Verification items for the finished model (mm, model axes). A direction names the side the tool comes from. Give positions to 0.01 mm unless a question says otherwise; leave off trailing zeros. Order: outer loops, then holes, each group sorted by start corner. A loop starts at its lowest first (then second) coordinate and runs counter-clockwise, first axis right, second up.
Autodesk Inventor part; units mm, degrees
ref_plane "YZ Plane" through (0, 0, 0) normal (1, 0, 0) x (0, 1, 0)
ref_plane "XZ Plane" through (0, 0, 0) normal (0, 1, 0) x (-1, 0, 0)
ref_plane "XY Plane" through (0, 0, 0) normal (0, 0, 1) x (1, 0, 0)
sketch "スケッチ1" plane through (0, 0, 0) normal (0, 0, 1) x (1, 0, 0)
  circle A0 centre (20, -42) radius 1
  circle A1 centre (4, -42) radius 1
  circle A2 centre (20, -6) radius 1
  circle A3 centre (20, -42) radius 1.1
  line L0 (22.5, -78.2) -> (22.5, -32.2)
  circle A4 centre (20, -42) radius 2.5
  circle A5 centre (20, -6) radius 2.5
  circle A6 centre (20, -6) radius 1.1
  circle A7 centre (4, -42) radius 1.1
  circle A8 centre (4, -42) radius 2.5
  line L1 (-8, -45.7) -> (-8, -64.7)
  line L2 (-8, -44.5) -> (-8, -39.5)
  line L3 (17.5, -42) -> (17.5, -6)
  line L4 (20, -39.5) -> (-8, -39.5)
  line L5 (20, -44.5) -> (4, -44.5)
  line L6 (4, -44.5) -> (-8, -44.5)
  line L7 (24, -24.4) -> (24, -30)
  line L8 (24, -32.2) -> (22.5, -32.2)
  line L9 (24, -22.2) -> (22.5, -22.2)
  line L10 (24, -32.2) -> (22.5, -32.2)
  line L11 (22.5, -32.2) -> (22.5, -22.2)
  line L12 (22.5, -22.2) -> (24, -22.2)
  line L13 (24, -22.2) -> (24, -32.2)
  line L14 (22.5, -22.2) -> (22.5, -6)
  line L15 (2, -43.5) -> (2, -4.5)
  arc A9 (2, -43.5) -> (2.5, -44) centre (2.5, -43.5) ccw
  line L16 (21.5, -44) -> (2.5, -44)
  arc A10 (21.5, -44) -> (22, -43.5) centre (21.5, -43.5) ccw
  line L17 (22, -4.5) -> (22, -43.5)
  arc A11 (22, -4.5) -> (21.5, -4) centre (21.5, -4.5) ccw
  line L18 (2.5, -4) -> (21.5, -4)
  arc A12 (2.5, -4) -> (2, -4.5) centre (2.5, -4.5) ccw
  line L19 (18.4286, -23.8214) -> (18.4286, -30.1786)
  line L20 (18.4286, -30.1786) -> (14.5714, -30.1786)
  line L21 (14.5714, -30.1786) -> (14.5714, -23.8214)
  line L22 (14.5714, -23.8214) -> (18.4286, -23.8214)
  circle A13 centre (12, -31.4) radius 1.1519
  line L23 (5.5714, -23.8214) -> (9.4286, -23.8214)
  line L24 (9.4286, -23.8214) -> (9.4286, -30.1786)
  line L25 (9.4286, -30.1786) -> (5.5714, -30.1786)
  line L26 (5.5714, -30.1786) -> (5.5714, -23.8214)
  circle A14 centre (20, -6) radius 1.8131
  circle A15 centre (4, -6) radius 1.8131
  circle A16 centre (20, -42) radius 1.8131
  circle A17 centre (4, -42) radius 1.8131
  arc A18 (18.25, -12.4893) -> (5.75, -12.5) centre (12, -12.5) ccw
  arc A19 (18.5, -12.25) -> (18.2502, -12.4893) centre (18.5, -12.5) ccw
  line L27 (18.5, -12.25) -> (20.25, -12.25)
  arc A20 (20.25, -12.75) -> (20.25, -12.25) centre (20.25, -12.5) ccw
  line L28 (20.25, -12.75) -> (18.5, -12.75)
  arc A21 (18.25, -12.5) -> (18.5, -12.75) centre (18.5, -12.5) ccw
  arc A22 (17.7742, -14.8918) -> (18.25, -12.5) centre (12, -12.5) ccw
  arc A23 (18.1009, -14.7565) -> (17.7742, -14.8918) centre (18.0052, -14.9874) ccw
  line L29 (18.1009, -14.7565) -> (19.7177, -15.4262)
  arc A24 (19.5263, -15.8881) -> (19.7177, -15.4262) centre (19.622, -15.6571) ccw
  line L30 (19.5263, -15.8881) -> (17.9095, -15.2184)
  arc A25 (17.7742, -14.8918) -> (17.9095, -15.2184) centre (18.0052, -14.9874) ccw
  arc A26 (16.4194, -16.9194) -> (17.7742, -14.8918) centre (12, -12.5) ccw
  arc A27 (16.773, -16.9194) -> (16.4194, -16.9194) centre (16.5962, -17.0962) ccw
  line L31 (16.773, -16.9194) -> (18.0104, -18.1569)
  arc A28 (17.6569, -18.5104) -> (18.0104, -18.1569) centre (17.8336, -18.3336) ccw
  line L32 (17.6569, -18.5104) -> (16.4194, -17.273)
  arc A29 (16.4194, -16.9194) -> (16.4194, -17.273) centre (16.5962, -17.0962) ccw
  arc A30 (14.3918, -18.2742) -> (16.4194, -16.9194) centre (12, -12.5) ccw
  arc A31 (14.7184, -18.4095) -> (14.3918, -18.2742) centre (14.4874, -18.5052) ccw
  line L33 (14.7184, -18.4095) -> (15.3881, -20.0263)
  arc A32 (14.9262, -20.2177) -> (15.3881, -20.0263) centre (15.1571, -20.122) ccw
  line L34 (14.9262, -20.2177) -> (14.2565, -18.6009)
  arc A33 (14.3918, -18.2742) -> (14.2565, -18.6009) centre (14.4874, -18.5052) ccw
  arc A34 (12, -18.75) -> (14.3918, -18.2742) centre (12, -12.5) ccw
  arc A35 (12.25, -19) -> (12, -18.75) centre (12, -19) ccw
  line L35 (12.25, -19) -> (12.25, -20.75)
  arc A36 (11.75, -20.75) -> (12.25, -20.75) centre (12, -20.75) ccw
  line L36 (11.75, -20.75) -> (11.75, -19)
  arc A37 (12, -18.75) -> (11.75, -19) centre (12, -19) ccw
  arc A38 (9.6082, -18.2742) -> (12, -18.75) centre (12, -12.5) ccw
  arc A39 (9.7435, -18.6009) -> (9.6082, -18.2742) centre (9.5126, -18.5052) ccw
  line L37 (9.7435, -18.6009) -> (9.0738, -20.2177)
  arc A40 (8.6119, -20.0263) -> (9.0738, -20.2177) centre (8.8429, -20.122) ccw
  line L38 (8.6119, -20.0263) -> (9.2816, -18.4095)
  arc A41 (9.6082, -18.2742) -> (9.2816, -18.4095) centre (9.5126, -18.5052) ccw
  arc A42 (7.5806, -16.9194) -> (9.6082, -18.2742) centre (12, -12.5) ccw
  arc A43 (7.5806, -17.273) -> (7.5806, -16.9194) centre (7.4038, -17.0962) ccw
  line L39 (7.5806, -17.273) -> (6.3431, -18.5104)
  arc A44 (5.9896, -18.1569) -> (6.3431, -18.5104) centre (6.1664, -18.3336) ccw
  line L40 (5.9896, -18.1569) -> (7.227, -16.9194)
  arc A45 (7.5806, -16.9194) -> (7.227, -16.9194) centre (7.4038, -17.0962) ccw
  arc A46 (6.2258, -14.8918) -> (7.5806, -16.9194) centre (12, -12.5) ccw
  arc A47 (6.0905, -15.2184) -> (6.2258, -14.8918) centre (5.9948, -14.9874) ccw
  line L41 (6.0905, -15.2184) -> (4.4737, -15.8881)
  arc A48 (4.2823, -15.4262) -> (4.4737, -15.8881) centre (4.378, -15.6571) ccw
  line L42 (4.2823, -15.4262) -> (5.8991, -14.7565)
  arc A49 (6.2258, -14.8918) -> (5.8991, -14.7565) centre (5.9948, -14.9874) ccw
  arc A50 (5.75, -12.5) -> (6.2258, -14.8918) centre (12, -12.5) ccw
  arc A51 (5.5, -12.75) -> (5.75, -12.5) centre (5.5, -12.5) ccw
  line L43 (5.5, -12.75) -> (3.75, -12.75)
  arc A52 (3.75, -12.25) -> (3.75, -12.75) centre (3.75, -12.5) ccw
  line L44 (3.75, -12.25) -> (5.5, -12.25)
  arc A53 (5.75, -12.5) -> (5.5, -12.25) centre (5.5, -12.5) ccw
  line L45 (18.9286, -30.6786) -> (18.9286, -23.3214)
  line L46 (18.9286, -23.3214) -> (14.0714, -23.3214)
  line L47 (14.0714, -23.3214) -> (14.0714, -30.6786)
  line L48 (14.0714, -30.6786) -> (18.9286, -30.6786)
  circle A54 centre (22.5, -21.1) radius 1.1
  circle A55 centre (22.5, -33.3) radius 1.1
  circle A56 centre (-9, -42) radius 1.1
  circle A57 centre (12, -12.5) radius 6.25
  circle A58 centre (12, -12.5) radius 8
  point P0 (0, 0)
  point P1 (-8, -42)
  point P2 (-8, -41.5417)
  point P3 (-8, -42.4583)
  point P4 (22.5, -42)
  point P5 (22.5, -34.4)
  point P6 (22.5, -20)
  point P7 (17.5, -9.5314)
  point P8 (18.25, -12.5)
  point P9 (17.5, -15.4686)
  point P10 (17.5, -17.6464)
  point P11 (17.5, -18.3536)
  point P12 (17.5, -23.3214)
  point P13 (17.5, -30.6786)
  point P14 (17.5, -39.5)
  point P15 (17.5, -6.6905)
  point P16 (17.5, -18.3095)
  dimension "d0" = 2.2
  dimension "d1" = 2.2
  dimension "d2" = 2.2
  dimension "d3" = 0.5
  dimension "d4" = 2.2
  dimension "d5" = 2.2
  dimension "d6" = 2.2
  dimension "d7" = 1
extrude "押し出し1" add sketch "スケッチ1" along normal blind 3 contours A4 L17 A55 L0 | A4 L17 | A4 L16 L17 | A4 L4 L3 L48 L45 L46 L32 A28 L31 A58 L30 A24 L29 L28 A20 L27 A5 L17 A54 A55 | L11 L9 L13 L7 L8 | A55 L17 A54 L11 | A4 L16 | A4 L3 L4 | L5 A8 L16 A4 | L16 A8 L4 L3 A4 | A54 L17 A5 L14 | L6 L2 A56 L4 L15 A8 A9 | A8 L16 | L16 A8 L15 | A8 L15 L4 | A5 L17 | A9 A8 | L15 A8 | L17 A5 A58 L18 | L18 A5 | A58 L3 A5 | L27 A20 L28 A58 | L3 A58 L31 A28 L32 | L29 A24 L30 A58 | A14 | A16 | A17
fillet "フィレット1" radius 2 4 edges at (17.5, -30.6786, 1.5) (18.9286, -30.6786, 1.5) (17.5, -23.3214, 1.5) (18.9286, -23.3214, 1.5)
sketch "スケッチ2" plane through (22.5, -42, 0) normal (1, 0, 0) x (0, 0, -1)
  circle A0 centre (-1.5, 24.8) radius 1.1
  circle A1 centre (-1.5, 4.8) radius 1.1
  point P0 (0, 42)
hole "穴1" at (22.5, -17.2, 1.5) at (22.5, -37.2, 1.5) direction (-1, 0, 0) diameter 1.567 depth 6.3 tip angle 118
sketch "スケッチ3" plane through (-8, -44.5, 0) normal (-1, 0, 0) x (0, 0, 1)
  line L0 (0, 2.5) -> (3, 2.5)
  point P0 (0, 44.5)
  point P1 (1.5, 2.5)
hole "穴2" at (-8, -42, 1.5) direction (1, 0, 0) diameter 1.567 depth 6.3 tip angle 118
fillet "フィレット2" radius 2 1 edges at (17.5, -39.5, 1.5)
properties part number "mata3" material "アルミニウム 2014-T4"
(1) Go/stop test with flat-tipped pins: pin 1 (0.9 mm diameter, centred on y = -35, z = 2, fed in from -X); pin 2 (1.5 mm diameter, centred on y = -15.5, z = 2, fed in from -X); pin 3 (0.9 mm diameter, centred on y = -15.5, z = 2, fed in from +X); pin 4 (1 mm diameter, centred on y = -32.5, z = 1.5, fed in from +X). Record where each tip stops, or that it passes through.
Solved:
pin 1: stops at x = 17.5
pin 2: stops at x = 19.07
pin 3: stops at x = 22.5
pin 4: stops at x = 24
(2) Release check for a two-part mould opening along X. For faces 1 (the flat face through (4, -39.5, 1)), 2 (the cylindrical face through (19.189, -42.743, 1.479)), 3 (the flat face through (18.929, -27, 1)) record: pulls with the +X half, pulls with the -X half, needs draft (parallel to the pull), parting line crosses it, or undercut.
Solved:
face 1: needs draft
face 2: undercut
face 3: pulls with the -X half
(3) Scan lines: line 1 (Z direction, x = -4, y = -42); line 2 (X direction, y = -43, z = 0.45); line 3 (Y direction, x = 5, z = 1.7). Record each from-to range of solid material in increasing order.
Solved:
line 1: z = 0 to 0.72, 2.28 to 3
line 2: x = -8 to 3.54, 4.46 to 19.54, 20.46 to 22.29
line 3: y = -44.5 to -42.46, -41.54 to -39.5
(4) Section check D-D, the plane y = -26. Enter the section's corners in (x, z), then the cut area to 3 significant figures.
Solved:
outline: (18.93, 0) - (24, 0) - (24, 3) - (18.93, 3) - close
area: 15.2 mm2
(5) Set-up check for faces 4 (the flat face through (22.5, -13, 1)), 5 (the cylindrical face through (4.59, -42.93, 1.48)), 6 (the flat face through (23, -32.2, 1)), 7 (the flat face through (17.5, -35, 1)), 8 (the flat face through (6, -44.5, 1)): record each of +Z, -Z, +X, -X, +Y, -Y from which the full face is reachable in a straight line by a thin tool's end or side.
Solved:
face 4: +Z, -Z, +X, +Y
face 5: +Z, -Z
face 6: +Z, -Z, +X, -Y
face 7: +Z, -Z, -X, +Y
face 8: +Z, -Z, +X, -X, -Y
(6) Section check B-B, the plane x = 20.5. Enter the section's corners in (y, z).
Solved:
outline: (-44.45, 0) - (-42.98, 0) - (-42.98, 3) - (-44.45, 3) - close; (-41.02, 0) - (-6.98, 0) - (-6.98, 3) - (-41.02, 3) - close; (-5.02, 0) - (-3.55, 0) - (-3.55, 3) - (-5.02, 3) - close; hole circle Ø1.57 at (-37.2, 1.5); hole circle Ø1.57 at (-17.2, 1.5)
(7) Section check A-A, the plane x = 4. Enter the section's corners in (y, z).
Solved:
outline: (-44.5, 0) - (-43.1, 0) - (-43.1, 3) - (-44.5, 3) - close; (-40.9, 0) - (-39.5, 0) - (-39.5, 3) - (-40.9, 3) - close
(8) Section check C-C, the plane y = -35. Enter the section's corners in (x, z), then the cut area to 3 significant figures.
Solved:
outline: (17.5, 0) - (22.5, 0) - (22.5, 3) - (17.5, 3) - close
area: 15.0 mm2
